from build123d import *

# Parameters (mm, degrees)
BOSS_EXTRUDE1_DEPTH     = 40
SKETCH2_W               = 55
SKETCH2_H               = 44
BOSS_EXTRUDE2_DEPTH     = 10
CUT_EXTRUDE2_DEPTH      = 65.807406984
CUT_EXTRUDE2_DEPTH_BACK = 65.807406984
SKETCH3_R               = 4.15
CUT_EXTRUDE3_DEPTH      = 65.807406984
CUT_EXTRUDE3_DEPTH_BACK = 65.807406984
SKETCH6_R               = 11.05
CUT_EXTRUDE4_DEPTH      = 60.718003985
FILLET1_R               = 2
FILLET2_R               = 1
SKETCH8_R               = 2
CUT_EXTRUDE5_DEPTH      = 56.532332924


with BuildPart() as part:
    # Sketch1 → Boss-Extrude1 (new, symmetric)
    with BuildSketch(Plane(origin=(0, 0, 0), x_dir=(0, 0, -1), z_dir=(1, 0, 0))):
        Polygon((-3, 6), (3, 6), (3, 4.1), (5.3, 4.1), (5.3, 2.48), (2.8, 0), (-2.8, 0), (-5.3, 2.48), (-5.3, 4.1), (-3, 4.1), align=None)
    extrude(amount=BOSS_EXTRUDE1_DEPTH, both=True)

    # Sketch2 → Boss-Extrude2 (add, symmetric)
    with BuildSketch(Plane.XY):
        with Locations((0, 28)):
            Rectangle(SKETCH2_W, SKETCH2_H)
    extrude(amount=BOSS_EXTRUDE2_DEPTH, both=True)

    # Sketch3 → Cut-Extrude2 (cut, two sides: drawn at the far end of the back side and taken through both)
    with BuildSketch(Plane.XY.offset(-CUT_EXTRUDE2_DEPTH_BACK)):
        with Locations((0, 27.15)):
            Circle(SKETCH3_R)
    extrude(amount=CUT_EXTRUDE2_DEPTH + CUT_EXTRUDE2_DEPTH_BACK, mode=Mode.SUBTRACT)

    # Sketch7 → Cut-Extrude3 (cut, two sides: drawn at the far end of the back side and taken through both)
    with BuildSketch(Plane.XY.offset(-CUT_EXTRUDE3_DEPTH_BACK)):
        with BuildLine():
            Line((27.5, 6), (14.560515369, 33.902324948))
            ThreePointArc((14.560515369, 33.902324948), (0, 43.2), (-14.560515369, 33.902324948))
            Line((-14.560515369, 33.902324948), (-27.5, 6))
            Line((-27.5, 6), (-40, 6))
            Line((-40, 6), (-40, 58.297822633))
            Line((-40, 58.297822633), (40, 58.297822633))
            Line((40, 58.297822633), (40, 6))
            Line((40, 6), (27.5, 6))
        make_face()
    extrude(amount=CUT_EXTRUDE3_DEPTH + CUT_EXTRUDE3_DEPTH_BACK, mode=Mode.SUBTRACT)

    # Sketch6 → Cut-Extrude4 (cut, through all)
    with BuildSketch(Plane.XY):
        with Locations((0, 27.15)):
            Circle(SKETCH6_R)
    extrude(amount=-CUT_EXTRUDE4_DEPTH, mode=Mode.SUBTRACT)

    # Fillet1
    fillet1_edges = [part.edges().sort_by_distance(p)[0] for p in [
        (21.030257684, 19.951162474, 10),
        (-21.030257684, 19.951162474, 10),
        (0, 43.2, 10),
        (21.030257684, 19.951162474, -10),
        (0, 43.2, -10),
        (-21.030257684, 19.951162474, -10),
    ]]
    fillet(fillet1_edges, radius=FILLET1_R)

    # Fillet2
    fillet2_edges = [part.edges().sort_by_distance(p)[0] for p in [
        (-4.15, 27.15, 10),
        (-4.15, 27.15, 0),
    ]]
    fillet(fillet2_edges, radius=FILLET2_R)

    # Sketch8 → Cut-Extrude5 (cut, through all)
    with BuildSketch(Plane(origin=(0, 6, 0), x_dir=(1, 0, 0), z_dir=(0, 1, 0))):
        with Locations(Location((35, 0, 0), (0, 0, 270))):
            Circle(SKETCH8_R)
        with Locations(Location((-35, 0, 0), (0, 0, 270))):
            Circle(SKETCH8_R)
    extrude(amount=-CUT_EXTRUDE5_DEPTH, mode=Mode.SUBTRACT)


solid = part.part
For this review, take the finished solid that the model builds, in its own axes (mm). A direction names the side the tool comes from. Give positions to 0.01 mm unless a question says otherwise; leave off trailing zeros. Loops run counter-clockwise (first coordinate to the right, second up) from the corner with the lowest first, then second, coordinate; pieces in that order, holes last.
Item 1: For line 1 along Y through (x, z) = (0, -4); line 2 along Y through (x, z) = (0, -6); line 3 along X through (y, z) = (2.9, 0), list the stretches that pass through material, from the lowest coordinate up.
Item 2: Take a section at B-B, the plane z = -1. State the section outline as (x, y) points.
Item 3: Draft analysis for pull direction X (two halves, no side actions). For faces 6 (the cylindrical face through (33, 3, 0)), 7 (the flat face through (1, 4.1, -4)), 8 (the cylindrical face through (20.6, 19.52, 9.4)), state which applies: +X half, -X half, draft (parallel to the pull), parting line (faces both ways), or undercut.
Item 4: Insertion check: pin 1 (2.5 mm diameter, centred on x = 35, z = 0, fed in from -Y); pin 2 (4.5 mm diameter, centred on x = -35, z = 0, fed in from +Y); pin 3 (2 mm diameter, centred on x = -26, z = 4, fed in from +Y); pin 4 (2.5 mm diameter, centred on x = 17, z = 4.5, fed in from +Y). Each pin has a flat end and moves straight along its axis. Give the tip position at first contact, or say it passes through.
Item 5: Take a section at D-D, the plane x = 0. State the section outline as (y, z) points, and give its area (3 significant figures).
Item 6: Tool access review of faces 1 (the flat face through (0, 6, 7)), 2 (the flat face through (0, 6, -6)), 3 (the flat face through (32, 6, 0)), 4 (the flat face through (1, 3, 5.3)), 5 (the flat face through (-32, 6, 0)): name each direction out of +Z, -Z, +X, -X, +Y, -Y from which nothing blocks a thin tool from reaching the whole face with its end or side.
Item 7: Take a section at C-C, the plane z = 4.5. State the section outline as (x, y) points.
Item 8: Take a section at A-A, the plane x = 35. State the section outline as (y, z) points.
Calculated:
1. line 1: y = 1.19 to 4.1, 6 to 16.1, 38.2 to 43.2
1. line 2: y = 6 to 16.1, 38.2 to 43.2
1. line 3: x = -40 to -37, -33 to 33, 37 to 40
2. outline: (-40, 0) - (-36.73, 0) - (-36.73, 6) - (-40, 6) - close; (-33.27, 0) - (33.27, 0) - (33.27, 6) - (27.5, 6) - (14.56, 33.9) arc R16.05 ccw to (-14.56, 33.9) - (-27.5, 6) - (-33.27, 6) - close; (36.73, 0) - (40, 0) - (40, 6) - (36.73, 6) - close; hole circle Ø22.1 at (0, 27.15)
3. face 6: undercut
3. face 7: draft
3. face 8: +X half
4. pin 1: passes through
4. pin 2: stops at y = 6
4. pin 3: stops at y = 11.39
4. pin 4: stops at y = 31.34
5. outline: (0, -2.8) - (2.48, -5.3) - (4.1, -5.3) - (4.1, -3) - (6, -3) - (6, -10) - (16.1, -10) - (16.1, 0) - (22, 0) arc R1 ccw to (23, 1) - (23, 9) arc R1 ccw to (22, 10) - (6, 10) - (6, 3) - (4.1, 3) - (4.1, 5.3) - (2.48, 5.3) - (0, 2.8) - close; (31.3, 1) arc R1 ccw to (32.3, 0) - (38.2, 0) - (38.2, -10) - (41.2, -10) arc R2 ccw to (43.2, -8) - (43.2, 8) arc R2 ccw to (41.2, 10) - (32.3, 10) arc R1 ccw to (31.3, 9) - close
5. area: 486 mm2
6. face 1: +Z, +X, -X
6. face 2: -Z, +X, -X
6. face 3: +Z, -Z, +X, +Y
6. face 4: +Z, +X, -X, -Y
6. face 5: +Z, -Z, -X, +Y
7. outline: (-40, 1.69) - (40, 1.69) - (40, 4.1) - (-40, 4.1) - close; (-27.5, 6) - (27.5, 6) - (14.56, 33.9) arc R16.05 ccw to (-14.56, 33.9) - close; hole circle Ø8.3 at (0, 27.15)
8. outline: (0, -2.8) - (2.48, -5.3) - (4.1, -5.3) - (4.1, -3) - (6, -3) - (6, -2) - (0, -2) - close; (0, 2) - (6, 2) - (6, 3) - (4.1, 3) - (4.1, 5.3) - (2.48, 5.3) - (0, 2.8) - close
